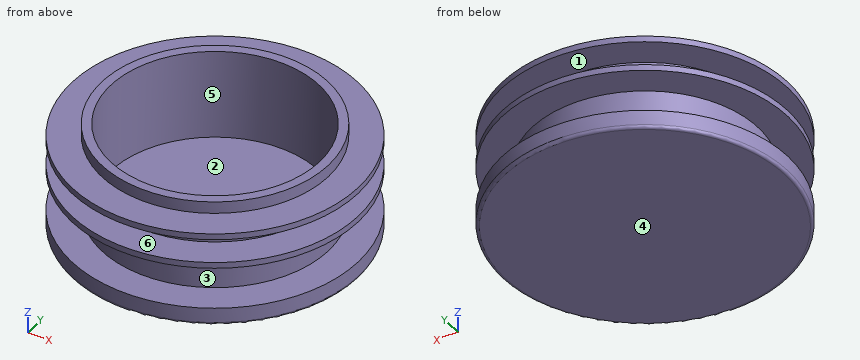
from build123d import *

# Parameters (mm, degrees)
SKETCH_R      = 24
PAD_DEPTH     = 3
SKETCH001_R   = 19
SKETCH001_R_2 = 17.5
PAD001_DEPTH  = 15
SKETCH002_R   = 24
SKETCH002_R_2 = 17.5
PAD002_DEPTH  = 1
SKETCH003_R   = 24
SKETCH003_R_2 = 17.5
PAD003_DEPTH  = 1
FILLET_R      = 0.5


with BuildPart() as part:
    # Sketch → Pad (new body)
    with BuildSketch(Plane.XY):
        Circle(SKETCH_R)
    extrude(amount=PAD_DEPTH)

    # Sketch001 (on Face3 of Pad) → Pad001 (join)
    with BuildSketch(Plane.XY.offset(3)):
        Circle(SKETCH001_R)
        Circle(SKETCH001_R_2, mode=Mode.SUBTRACT)
    extrude(amount=PAD001_DEPTH)

    # Sketch002 (on DatumPlane) → Pad002 (join)
    with BuildSketch(Plane.XY.offset(10)):
        Circle(SKETCH002_R)
        Circle(SKETCH002_R_2, mode=Mode.SUBTRACT)
    extrude(amount=PAD002_DEPTH)

    # Sketch003 (on DatumPlane) → Pad003 (join)
    with BuildSketch(Plane.XY.offset(15)):
        Circle(SKETCH003_R)
        Circle(SKETCH003_R_2, mode=Mode.SUBTRACT)
    extrude(amount=PAD003_DEPTH)

    # Fillet
    fillet_edges = [part.edges().sort_by_distance(p)[0] for p in [
        (-24, 0, 0),
    ]]
    fillet(fillet_edges, radius=FILLET_R)


solid = part.part
Read the model definition and answer for the solid it produces. Units are mm, in the model's axes. Face numbers are marked on the shaded views. A direction names the side the tool comes from. Coordinates: 2 decimals unless noted, no trailing zeros. Order: outer loops, then holes, each group sorted by start corner. A loop starts at its lowest first (then second) coordinate and runs counter-clockwise, first axis right, second up. Notation, with made-up numbers: (-23.75, 51) -> (25.25, 51) arc R32 ccw to (25.25, 86) -> close; hole circle Ø11 at (19.25, 74). An arc over 180 degrees is marked (long way). Answer as a JSON object with one key per item and string values.
1) Each of these flat-tipped pins is pushed along its axis until it touches: pin 1 (1 mm diameter, centred on x = -16.5, y = -11, fed in from -Z); pin 2 (17.5 mm diameter, centred on x = 1, y = 4, fed in from +Z); pin 3 (1.5 mm diameter, centred on x = 13, z = 4, fed in from +Y); pin 4 (1.5 mm diameter, centred on y = -12.5, z = 10.5, fed in from -X). Where does it stop, or does it pass through?
Model answer:
{"pin 1": "stops at z = 0", "pin 2": "stops at z = 3", "pin 3": "stops at y = 14.52", "pin 4": "stops at x = -20.93"}
2) The mould has two halves that part along Y. Classify the marked faces 1, 2 and 3: released by +Y, released by -Y, zero draft, split by the parting line, or undercut.
Model answer:
{"face 1": "zero draft", "face 2": "undercut", "face 3": "split by the parting line"}
3) A tool of negligible diameter and unlimited length cuts with its end or side. For the marked faces 4, 5 and 6, from which of +Z, -Z, +X, -X, +Y, -Y can it reach the whole face along a straight path? Write none if from no direction.
Model answer:
{"face 4": "-Z, +X, -X, +Y, -Y", "face 5": "+Z", "face 6": "none"}
4) A cutting plane is placed at C-C, the plane z = 4. Determine the outline of the cut face in (x, y).
Model answer:
{"outline": "circle Ø38 at (0, 0); hole circle Ø35 at (0, 0)"}
5) Consider line 1 along Z through (x, y) = (-16, -15.5); line 2 along Y through (x, z) = (0, 14); line 3 along Y through (x, z) = (0, 10.5). Determine where each line is inside the solid, lowest interval first. Write a range as from..to.
Model answer:
{"line 1": "z = 0..3, 10..11, 15..16", "line 2": "y = -19..-17.5, 17.5..19", "line 3": "y = -24..-17.5, 17.5..24"}
